The drawing under review shows one solid part. Ordinate dimensions are in mm from its lowest x, y, z. A direction names the side the tool comes from. Round coordinates to 2 decimals unless told otherwise and drop trailing zeros. Order: outer loops, then holes, each group sorted by start corner. A loop starts at its lowest first (then second) coordinate and runs counter-clockwise, first axis right, second up.
1) To check wall thickness, follow L1, parallel to Z at x = 31.5, y = 11.5; L2, parallel to X at y = 15, z = 62.9; L3, parallel to Y at x = 17, z = 57. State the ranges of each line that lie inside material, in increasing order.
2) Consider section A-A (y = 20.5). Give the boundary of the cut face in (x, z), then the cut area to 3 significant figures.
3) Clearance check with flat-ended pins moving along their axes: P1, Ø2.5, axis at x = 35, y = 15, coming from the -Z side; P2, Ø24, axis at x = 37, z = 42.5, coming from the +Y side. State where each tip first meets the part, or that it passes through.
4) Consider section D-D (x = 24.5). Give the boundary of the cut face in (y, z).
5) Machinability: for the marked faces 1 and 2, which of the approach directions +Z, -Z, +X, -X, +Y, -Y give a long, thin tool a straight path to every point of the face, cutting with its end or side? Answer none if there is none.
6) Consider section B-B (x = 35). Give the number of separate pieces and of enclosed holes in the cut face, then the cut area to 4 significant figures.
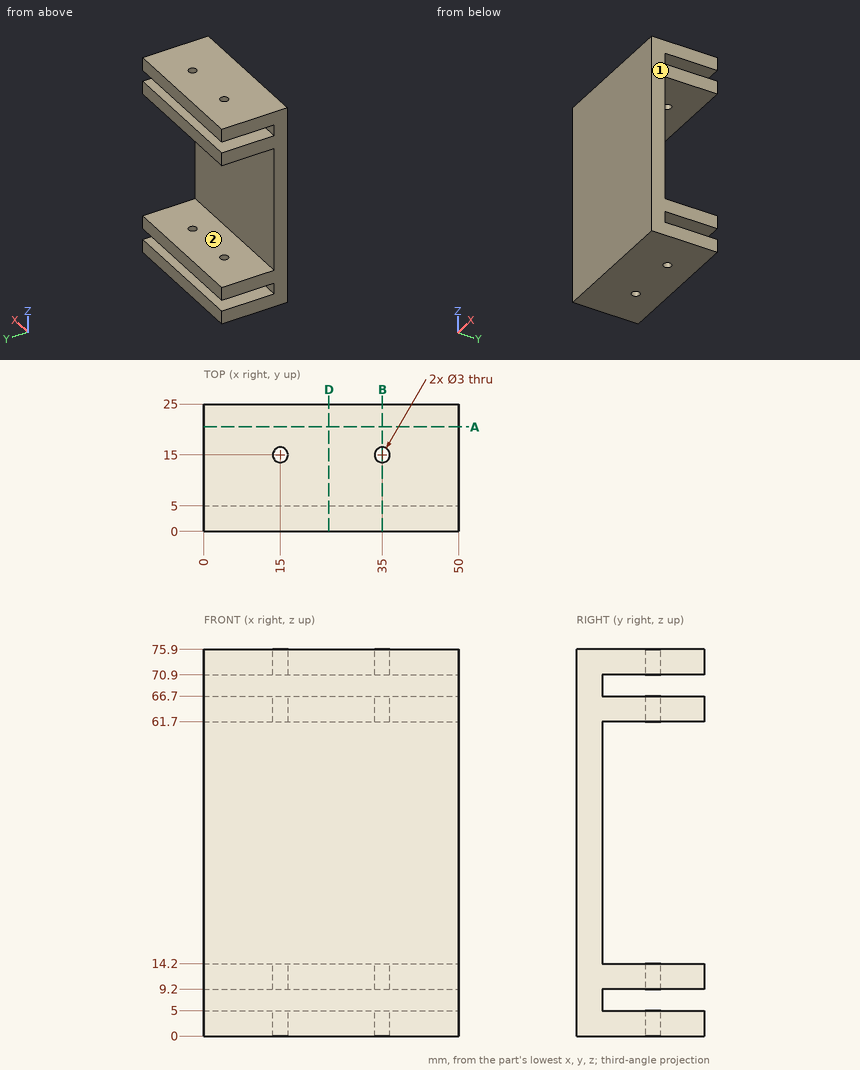
Answer below:
1. L1: z = 0 to 5, 9.2 to 14.2, 61.7 to 66.7, 70.9 to 75.9
1. L2: x = 0 to 13.5, 16.5 to 33.5, 36.5 to 50
1. L3: y = 0 to 5
2. outline: (0, 0) - (50, 0) - (50, 5) - (0, 5) - close; (0, 9.2) - (50, 9.2) - (50, 14.2) - (0, 14.2) - close; (0, 61.7) - (50, 61.7) - (50, 66.7) - (0, 66.7) - close; (0, 70.9) - (50, 70.9) - (50, 75.9) - (0, 75.9) - close
2. area: 1,000 mm2
3. P1: passes through
3. P2: stops at y = 5
4. outline: (0, 0) - (25, 0) - (25, 5) - (5, 5) - (5, 9.2) - (25, 9.2) - (25, 14.2) - (5, 14.2) - (5, 61.7) - (25, 61.7) - (25, 66.7) - (5, 66.7) - (5, 70.9) - (25, 70.9) - (25, 75.9) - (0, 75.9) - close
5. face 1: +Z, -Z, +X, +Y, -Y
5. face 2: +X, -X, +Y
6. separate pieces: 5
6. enclosed holes: 0
6. area: 719.5 mm2
